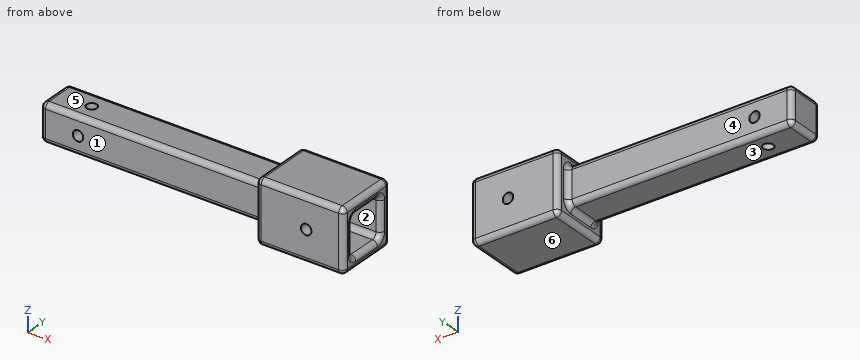
from build123d import *

# Parameters (mm, degrees)
SKETCH1_W                = 90
SKETCH1_H                = 15
BOSS_EXTRUDE1_DEPTH      = 7.5
BOSS_EXTRUDE1_DEPTH_BACK = 7.5
BOSS_EXTRUDE2_DEPTH      = 12.5
BOSS_EXTRUDE2_DEPTH_BACK = 12.5
SKETCH3_R                = 2.1
CUT_EXTRUDE1_DEPTH       = 21
SKETCH5_R                = 2.1
CUT_EXTRUDE3_DEPTH       = 26
SKETCH6_W                = 15.8
SKETCH6_H                = 15.8
CUT_EXTRUDE4_DEPTH       = 32
SKETCH8_R                = 2.1
CUT_EXTRUDE5_DEPTH       = 21
FILLET1_R                = 2


with BuildPart() as part:
    # Sketch1 → Boss-Extrude1 (new body, two sides)
    with BuildSketch(Plane(origin=(0, 0, 0), x_dir=(1, 0, 0), z_dir=(0, 1, 0))) as boss_extrude1_sk:
        with Locations((45, -7.5)):
            Rectangle(SKETCH1_W, SKETCH1_H)
    extrude(amount=BOSS_EXTRUDE1_DEPTH)
    extrude(boss_extrude1_sk.sketch, amount=-BOSS_EXTRUDE1_DEPTH_BACK)

    # Sketch1_3 → Boss-Extrude2 (add, two sides)
    with BuildSketch(Plane(origin=(0, 0, 0), x_dir=(1, 0, 0), z_dir=(0, 1, 0))) as boss_extrude2_sk:
        Polygon((125, 5), (125, -20), (90, -20), (90, -15), (90, 0), (90, 5), align=None)
    extrude(amount=BOSS_EXTRUDE2_DEPTH)
    extrude(boss_extrude2_sk.sketch, amount=-BOSS_EXTRUDE2_DEPTH_BACK)

    # Sketch3 → Cut-Extrude1 (cut, through all)
    with BuildSketch(Plane.XY.offset(15)):
        with Locations((15, 0)):
            Circle(SKETCH3_R)
    extrude(amount=-CUT_EXTRUDE1_DEPTH, mode=Mode.SUBTRACT)

    # Sketch5 → Cut-Extrude3 (cut, through all)
    with BuildSketch(Plane(origin=(0, 12.5, 0), x_dir=(1, 0, 0), z_dir=(0, 1, 0))):
        with Locations((110, -7.5)):
            Circle(SKETCH5_R)
    extrude(amount=-CUT_EXTRUDE3_DEPTH, mode=Mode.SUBTRACT)

    # Sketch6 → Cut-Extrude4 (cut)
    with BuildSketch(Plane(origin=(125, 0, 0), x_dir=(0, 0, -1), z_dir=(1, 0, 0))):
        with Locations((-7.5, 0)):
            Rectangle(SKETCH6_W, SKETCH6_H)
    extrude(amount=-CUT_EXTRUDE4_DEPTH, mode=Mode.SUBTRACT)

    # Sketch8 → Cut-Extrude5 (cut, through all)
    with BuildSketch(Plane.XZ.offset(7.5)):
        with Locations((15, 7.5)):
            Circle(SKETCH8_R)
    extrude(amount=-CUT_EXTRUDE5_DEPTH, mode=Mode.SUBTRACT)

    # Fillet1
    fillet1_edges = [part.edges().sort_by_distance(p)[0] for p in [
        (45, -7.5, 0),
        (90, 7.5, 7.5),
        (45, 7.5, 0),
        (0, -7.5, 7.5),
        (0, 7.5, 7.5),
        (45, 7.5, 15),
        (45, -7.5, 15),
        (90, 0, 20),
        (90, -12.5, 7.5),
        (125, 0, -5),
        (125, 12.5, 7.5),
        (125, 0, 20),
        (107.5, -12.5, 20),
        (90, 0, -5),
        (107.5, 12.5, -5),
        (125, -12.5, 7.5),
        (107.5, -12.5, -5),
        (90, 12.5, 7.5),
        (107.5, 12.5, 20),
        (90, -7.5, 7.5),
        (93, 7.9, 7.5),
        (109, 7.9, 15.4),
        (93, -7.9, 7.5),
        (109, -7.9, -0.4),
        (93, 0, 15.4),
        (109, -7.9, 15.4),
        (93, 0, -0.4),
        (109, 7.9, -0.4),
        (125, 0, 15.4),
        (125, -7.9, 7.5),
        (125, 0, -0.4),
        (125, 7.9, 7.5),
        (90, 0, 15),
        (0, 0, 15),
        (0, 0, 0),
        (90, 0, 0),
    ]]
    fillet(fillet1_edges, radius=FILLET1_R)


solid = part.part
Geometry check sheet. Reference: the model listing, model coordinates, mm. Face numbers are marked on the shaded views. A direction names the side the tool comes from. Round coordinates to 2 decimals unless told otherwise and drop trailing zeros. Loops run counter-clockwise (first coordinate to the right, second up) from the corner with the lowest first, then second, coordinate; pieces in that order, holes last.
Item 1: Mould release check, pull along Z, two halves, no side actions. Record for the marked faces 1, 2 and 3: pulls with the +Z half, pulls with the -Z half, needs draft (parallel to the pull), parting line crosses it, or undercut.
Item 2: Thickness scan on line 1 (Y direction, x = 95, z = 13.25); line 2 (X direction, y = -1.75, z = 7.5); line 3 (Y direction, x = 86.5, z = 8.75). Record the ranges inside material, lowest first.
Item 3: Gauge pin test, flat ends, axial feed: pin 1 (3.5 mm diameter, centred on x = 15, y = 0, fed in from +Z); pin 2 (12 mm diameter, centred on x = 32, y = 1.5, fed in from -Z); pin 3 (4 mm diameter, centred on x = 60, z = 4.5, fed in from -Y); pin 4 (12 mm diameter, centred on x = 66.5, y = -1, fed in from +Z). Record the tip position at first contact, or that the pin passes through.
Item 4: Cross-section at C-C on x = 110. Record the boundary of the cut face in (y, z), then the cut area to 3 significant figures.
Item 5: Access from +Z, -Z, +X, -X, +Y, -Y to the whole of each face (thin tool, end or side, straight path). Record for the marked faces 4, 5 and 6.
Item 6: Cross-section at B-B on z = 4.25. Record the boundary of the cut face in (x, y), then the cut area to 3 significant figures.
Item 7: Cross-section at A-A on x = 15. Record the boundary of the cut face in (y, z).
Item 8: Cross-section at D-D on x = 41.5. Record the boundary of the cut face in (y, z).
Answer sheet:
1. face 1: needs draft
1. face 2: undercut
1. face 3: pulls with the -Z half
2. line 1: y = -12.5 to -7.9, 7.9 to 12.5
2. line 2: x = 0 to 12.9, 17.1 to 93
2. line 3: y = -7.5 to 7.5
3. pin 1: passes through
3. pin 2: stops at z = 0
3. pin 3: stops at y = -7.5
3. pin 4: stops at z = 15
4. outline: (-12.5, -3) arc R2 ccw to (-10.5, -5) - (10.5, -5) arc R2 ccw to (12.5, -3) - (12.5, 5.4) - (7.9, 5.4) - (7.9, 1.6) arc R2 cw to (5.9, -0.4) - (-5.9, -0.4) arc R2 cw to (-7.9, 1.6) - (-7.9, 5.4) - (-12.5, 5.4) - close; (-12.5, 9.6) - (-7.9, 9.6) - (-7.9, 13.4) arc R2 cw to (-5.9, 15.4) - (5.9, 15.4) arc R2 cw to (7.9, 13.4) - (7.9, 9.6) - (12.5, 9.6) - (12.5, 18) arc R2 ccw to (10.5, 20) - (-10.5, 20) arc R2 ccw to (-12.5, 18) - close
4. area: 337 mm2
5. face 4: +Z, -Z, -X, +Y
5. face 5: +Z, -X, +Y, -Y
5. face 6: -Z, +X, -X, +Y, -Y
6. outline: (0, -5.5) arc R2 ccw to (2, -7.5) - (88, -7.5) arc R2 cw to (90, -9.5) - (90, -10.5) arc R2 ccw to (92, -12.5) - (123, -12.5) arc R2 ccw to (125, -10.5) - (125, -9.9) arc R2 ccw to (123, -7.9) - (95, -7.9) arc R2 cw to (93, -5.9) - (93, 5.9) arc R2 cw to (95, 7.9) - (123, 7.9) arc R2 ccw to (125, 9.9) - (125, 10.5) arc R2 ccw to (123, 12.5) - (92, 12.5) arc R2 ccw to (90, 10.5) - (90, 9.5) arc R2 cw to (88, 7.5) - (2, 7.5) arc R2 ccw to (0, 5.5) - close; hole circle Ø4.2 at (15, 0)
6. area: 1,700 mm2
7. outline: (-7.5, 2) arc R2 ccw to (-5.5, 0) - (-2.1, 0) - (-2.1, 5.4) - (-7.5, 5.4) - close; (-7.5, 9.6) - (-2.1, 9.6) - (-2.1, 15) - (-5.5, 15) arc R2 ccw to (-7.5, 13) - close; (2.1, 0) - (5.5, 0) arc R2 ccw to (7.5, 2) - (7.5, 5.4) - (2.1, 5.4) - close; (2.1, 9.6) - (7.5, 9.6) - (7.5, 13) arc R2 ccw to (5.5, 15) - (2.1, 15) - close
8. outline: (-7.5, 2) arc R2 ccw to (-5.5, 0) - (5.5, 0) arc R2 ccw to (7.5, 2) - (7.5, 13) arc R2 ccw to (5.5, 15) - (-5.5, 15) arc R2 ccw to (-7.5, 13) - close
